from build123d import *

# Parameters (mm, degrees)
F0_W     = 1066.8
F0_H     = 666.75
F0_R     = 12.7
F0_R_2   = 6.35
F0_W_2   = 76.2
F0_H_2   = 546.1
F1_DEPTH = 18.542


with BuildPart() as f1:
    # F0 (on Front) → F1 (new body)
    with BuildSketch(Plane.XZ):
        with Locations((0, 3.175)):
            Rectangle(F0_W, F0_H)
        with Locations((-482.6, -279.4)):
            Circle(F0_R, mode=Mode.SUBTRACT)
        with Locations((482.6, -279.4)):
            Circle(F0_R, mode=Mode.SUBTRACT)
        with Locations((0, -127)):
            Circle(F0_R_2, mode=Mode.SUBTRACT)
        with Locations((-368.3, 6.35)):
            Rectangle(F0_W_2, F0_H_2, mode=Mode.SUBTRACT)
        with Locations((368.3, 6.35)):
            Rectangle(F0_W_2, F0_H_2, mode=Mode.SUBTRACT)
    extrude(amount=F1_DEPTH)


solid = f1.part
Work out the finished part from the listing and answer in its coordinate system (mm). Round coordinates to 2 decimals unless told otherwise and drop trailing zeros. Write each loop counter-clockwise with the first axis right and the second up, starting at its lowest first coordinate (ties: lowest second). Pieces come first, ordered by that corner, then holes. Notation, with made-up numbers: M -35.75,-19 L -18.75,-19 A15 cw -18.75,6 Z; hole C 88,77 d8. An arc over 180 degrees is marked long. Use a Markdown table: item, result.
1) The part is cut by section B-B on y = -12.75. Give the vertices of the cut face in (x, z).
Taken from the geometry:
| item | result |
|---|---|
| outline | M -533.4,-330.2 L 533.4,-330.2 L 533.4,336.55 L -533.4,336.55 Z; hole C -482.6,-279.4 d25.4; hole M -406.4,-266.7 L -330.2,-266.7 L -330.2,279.4 L -406.4,279.4 Z; hole C 0,-127 d12.7; hole M 330.2,-266.7 L 406.4,-266.7 L 406.4,279.4 L 330.2,279.4 Z; hole C 482.6,-279.4 d25.4 |
2) Determine the mould class of faces 1 (the face through (-7, 0, 8)), 2 (the face through (488.46, -9.141, -290.667)) for opening direction X: pulls with the +X half, pulls with the -X half, needs draft (parallel to the pull), parting line crosses it, or undercut.
Taken from the geometry:
| item | result |
|---|---|
| face 1 | needs draft |
| face 2 | undercut |
3) Flat-ended cylindrical pins translate along their axes: pin 1 (15 mm diameter, centred on x = 482.6, z = -279.4, fed in from -Y); pin 2 (1.5 mm diameter, centred on x = 412, z = -171, fed in from +Y). Find the tip coordinate at first contact, or state that the pin passes through.
Taken from the geometry:
| item | result |
|---|---|
| pin 1 | passes through |
| pin 2 | stops at y = 0 |
4) The part is cut by section A-A on z = -279.4. Give the vertices of the cut face in (x, y).
Taken from the geometry:
| item | result |
|---|---|
| outline | M -533.4,-18.54 L -495.3,-18.54 L -495.3,0 L -533.4,0 Z; M -469.9,-18.54 L 469.9,-18.54 L 469.9,0 L -469.9,0 Z; M 495.3,-18.54 L 533.4,-18.54 L 533.4,0 L 495.3,0 Z |
5) Consider line 1 (X direction, y = -15.25, z = -265); line 2 (Z direction, x = -351, y = -4.25); line 3 (Z direction, x = 0, y = -12.5). Determine where each line is inside the solid, lowest interval first. Write a range as [from, to].
Taken from the geometry:
| item | result |
|---|---|
| line 1 | x = [-533.4, -406.4], [-330.2, 330.2], [406.4, 533.4] |
| line 2 | z = [-330.2, -266.7], [279.4, 336.55] |
| line 3 | z = [-330.2, -133.35], [-120.65, 336.55] |
6) The part is cut by section C-C on x = 482.6. Give the vertices of the cut face in (y, z).
Taken from the geometry:
| item | result |
|---|---|
| outline | M -18.54,-330.2 L 0,-330.2 L 0,-292.1 L -18.54,-292.1 Z; M -18.54,-266.7 L 0,-266.7 L 0,336.55 L -18.54,336.55 Z |
7) The part is cut by section D-D on z = 110.5. Give the vertices of the cut face in (x, y).
Taken from the geometry:
| item | result |
|---|---|
| outline | M -533.4,-18.54 L -406.4,-18.54 L -406.4,0 L -533.4,0 Z; M -330.2,-18.54 L 330.2,-18.54 L 330.2,0 L -330.2,0 Z; M 406.4,-18.54 L 533.4,-18.54 L 533.4,0 L 406.4,0 Z |
